Verification items for the finished model (mm, model axes). Give positions to 0.01 mm unless a question says otherwise; leave off trailing zeros. Loops run counter-clockwise (first coordinate to the right, second up) from the corner with the lowest first, then second, coordinate; pieces in that order, holes last. Notation, with made-up numbers: (8, 74) - (42, 74) arc R36 ccw to (42, 112) - close; hole circle Ø7 at (62.25, -37). An arc over 180 degrees is marked (long way). Put each result on its own line as item: value. Start each with the question number.
```python
from build123d import *

# Parameters (mm, degrees)
F0_R            = 7.62
F1_DEPTH        = 7.62
F2_R            = 0.635
F3_DEPTH        = 15.24
F5_DEPTH        = 15.24
F5_COPIES_COUNT = 30


# Not quite as in the source:
# - a pattern or mirror of a feature is missing from the dataset's text; its kind, count and spacing are read off the source's solid


with BuildPart() as f1:
    # F0 (on Top) → F1 (new body, symmetric)
    with BuildSketch(Plane.XY):
        Circle(F0_R)
    extrude(amount=F1_DEPTH, both=True)

    # F2 (on face) → F3 (cut, through all)
    with BuildSketch(Plane.XY.offset(7.62)):
        Circle(F2_R)
    extrude(amount=-F3_DEPTH, mode=Mode.SUBTRACT)

    # F4 (on face) → F5 (cut, through all)
    with BuildSketch(Plane.XY.offset(7.62)):
        with BuildLine():
            ThreePointArc((1.20963125, 7.5233763856), (0.7965068901, 7.5782568427), (0.381, 7.6104690394))
            Line((0.381, 7.6104690394), (0.508, 6.3296473835))
            ThreePointArc((0.508, 6.3296473835), (0.6637557417, 6.3152140356), (0.8191087086, 6.2969485406))
            Line((0.8191087086, 6.2969485406), (1.20963125, 7.5233763856))
        make_face()
    f5 = extrude(amount=-F5_DEPTH, mode=Mode.SUBTRACT)

    # F5_copies: F5 ×30 about axis
    f5_copies_axis = Axis((0, 0, 0), (0, 0, 1))
    for i in range(1, F5_COPIES_COUNT):
        add(f5.rotate(f5_copies_axis, i * 360 / F5_COPIES_COUNT), mode=Mode.SUBTRACT)


solid = f1.part
```
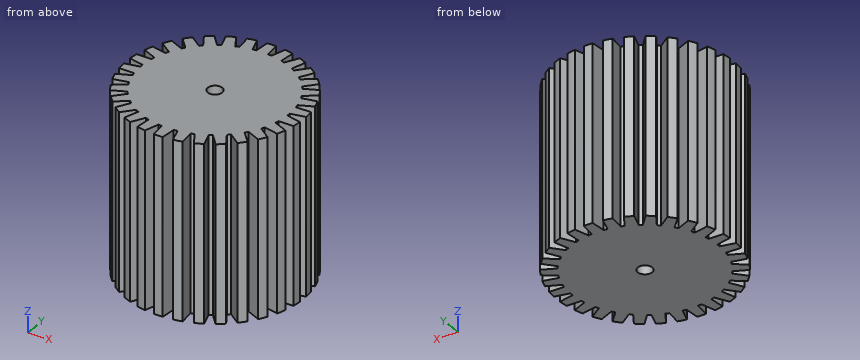
1) Depth check by flat-ended pin: P1, Ø5, axis at y = 1, z = 5, coming from the -X side; P2, Ø5, axis at x = 4.5, z = 0.5, coming from the +Y side; P3, Ø2, axis at y = -3, z = -1.5, coming from the +X side. Enter the tip coordinate at first touch or a pass-through.
2) Section check A-A, the plane x = 0. Enter the section's corners in (y, z) (3 decimals).
3) Scan lines: line 1 along Y through (x, z) = (5.5, 1.75); line 2 along X through (y, z) = (6.5, 0.5); line 3 along Y through (x, z) = (-6, -5.5). Record each from-to range of solid material in increasing order. Write a range as from..to.
Results are:
1. P1: stops at x = -7.61
1. P2: stops at y = 7.11
1. P3: stops at x = 7.35
2. outline: (-7.62, -7.62) - (-0.635, -7.62) - (-0.635, 7.62) - (-7.62, 7.62) - close; (0.635, -7.62) - (7.62, -7.62) - (7.62, 7.62) - (0.635, 7.62) - close
3. line 1: y = -5.27..-4.36, -3.73..3.73, 4.36..5.27
3. line 2: x = -3.34..-2.4, -1.86..-0.88, -0.49..0.49, 0.88..1.86, 2.4..3.34
3. line 3: y = -3.95..-2.91, -2.47..2.47, 2.91..3.95
